from build123d import *

# Parameters (mm, degrees)
F1_DEPTH = 18


with BuildPart() as f1:
    # F0 (on Front) → F1 (new body)
    with BuildSketch(Plane.XZ):
        with BuildLine():
            Line((-494.9431181919, -380.3196549416), (-495.3364644899, -390.3106509103))
            Line((-495.3364644899, -390.3106509103), (-474.3992558025, -390.3106509103))
            Line((-474.3992558025, -390.3106509103), (-442.9078605118, -13.6198989728))
            ThreePointArc((-442.9078605118, -13.6198989728), (-445.4387975319, -5.6995339283), (-438.0486109698, -9.5104350311))
            Line((-438.0486109698, -9.5104350311), (-429.079897486, -10.2602206314))
            ThreePointArc((-429.079897486, -10.2602206314), (-421.1595324415, -7.7292836113), (-424.9704335443, -15.1194701734))
            Line((-424.9704335443, -15.1194701734), (-456.3364644899, -390.3106509103))
            Line((-456.3364644899, -390.3106509103), (-435.3364644899, -390.3106509103))
            Line((-435.3364644899, -390.3106509103), (-349.9298685588, 255.9864675478))
            ThreePointArc((-349.9298685588, 255.9864675478), (-336.6411341811, 280.8261308929), (-310.274619413, 290.7461225986))
            Line((-310.274619413, 290.7461225986), (-55.3364644899, 290.7461225986))
            ThreePointArc((-55.3364644899, 290.7461225986), (-27.0287216569, 302.4853424307), (-15.3365196272, 330.8125378136))
            Line((-15.3365196272, 330.8125378136), (-15.4040666505, 371.4941377938))
            Line((-15.4040666505, 371.4941377938), (-26.1865943467, 371.4941377938))
            Line((-26.1865943467, 371.4941377938), (-26.4555723936, 385.8212303749))
            Line((-26.4555723936, 385.8212303749), (-26.474497292, 389.6893490897))
            Line((-26.474497292, 389.6893490897), (-44.4864644899, 389.6893490897))
            Line((-44.4864644899, 389.6893490897), (-44.4864644899, 371.4941377938))
            Line((-44.4864644899, 371.4941377938), (-55.3364644899, 371.4941377938))
            Line((-55.3364644899, 371.4941377938), (-55.3364644899, 327.1893490897))
            ThreePointArc((-55.3364644899, 327.1893490897), (-57.533163631, 321.8860482309), (-62.8364644899, 319.6893490897))
            ThreePointArc((-62.8364644899, 319.6893490897), (-68.1397653488, 321.8860482309), (-70.3364644899, 327.1893490897))
            Line((-70.3364644899, 327.1893490897), (-70.3364644899, 389.6893490897))
            Line((-70.3364644899, 389.6893490897), (-83.3364644899, 389.6893490897))
            add(Edge.make_bspline(
                [(-83.3364644899, 389.6893490897), (-86.0423866242, 388.9113420461), (-91.2893973468, 387.4027209189), (-94.0159938946, 383.2265543698), (-95.3364644899, 381.2040677155)],
                knots=[0, 0, 0, 0, 0.5157073765, 1, 1, 1, 1], degree=3))
            Line((-95.3364644899, 381.2040677155), (-80.3364644899, 381.2289734555))
            Line((-80.3364644899, 381.2289734555), (-80.3364644899, 327.1893490897))
            ThreePointArc((-80.3364644899, 327.1893490897), (-82.533163631, 321.8860482309), (-87.8364644899, 319.6893490897))
            ThreePointArc((-87.8364644899, 319.6893490897), (-93.1397653488, 321.8860482309), (-95.3364644899, 327.1893490897))
            Line((-95.3364644899, 327.1893490897), (-95.3364644899, 370.6893490897))
            Line((-95.3364644899, 370.6893490897), (-95.3364644899, 371.6893490897))
            Line((-95.3364644899, 371.6893490897), (-435.3364644899, 371.6893490897))
            Line((-435.3364644899, 371.6893490897), (-435.3364644899, 375.1893490897))
            Line((-435.3364644899, 375.1893490897), (-435.3364644899, 376.1893490897))
            Line((-435.3364644899, 376.1893490897), (-435.3364644899, 380.6893490897))
            Line((-435.3364644899, 380.6893490897), (-405.3364644899, 380.6893490897))
            Line((-405.3364644899, 380.6893490897), (-405.3364644899, 389.6893490897))
            Line((-405.3364644899, 389.6893490897), (-445.3364644899, 389.6893490897))
            add(Edge.make_bspline(
                [(-445.3364644899, 389.6893490897), (-450.2049500524, 389.0615823794), (-459.5920285383, 387.2680457186), (-463.5495128465, 378.4364704972), (-465.3198116993, 372.6887939967)],
                knots=[0, 0, 0, 0, 0.4865626406, 1, 1, 1, 1], degree=3))
            Line((-465.3198116993, 372.6887939967), (-465.3905866055, 370.3146473532))
            Line((-465.3905866055, 370.3146473532), (-494.9431181919, -380.3196549416))
        make_face()
    extrude(amount=F1_DEPTH)


solid = f1.part
The listing builds one solid part. Answer for the finished solid, in the listing's coordinates (mm). A direction names the side the tool comes from. Coordinates: 2 decimals unless noted, no trailing zeros. Write each loop counter-clockwise with the first axis right and the second up, starting at its lowest first coordinate (ties: lowest second). Pieces come first, ordered by that corner, then holes. Notation, with made-up numbers: (-32.5, 0) - (-4.5, 0) arc R27 cw to (-4.5, 19) - close; hole circle Ø3 at (-16.5, -21.75). An arc over 180 degrees is marked (long way). Answer as CSV lines item,"result".
1. Determine the mould class of faces 1 (the flat face through (-425, -9, 389.689)), 2 (the flat face through (-393.23, -8.87, -71.69)), 3 (the flat face through (-44.486, -9, 381)) for opening direction X: +X half, -X half, draft (parallel to the pull), parting line (faces both ways), or undercut.
Computed values:
face 1,"draft"
face 2,"+X half"
face 3,"undercut"
2. Given P1, Ø6, axis at y = -4, z = -191.5, coming from the +X side; P2, Ø2.5, axis at y = -9.5, z = 376, coming from the +X side; P3, Ø5.5, axis at x = -20, y = -8.5, coming from the +Z side, each flat-ended and moving along its own axis, determine where each tip first touches the part or whether it passes through.
Computed values:
P1,"stops at x = -408.67"
P2,"stops at x = -26.25"
P3,"stops at z = 371.49"
3. Find section C-C (z = -294.5). Give the vertices of the cut face in (x, y).
Computed values:
outline,"(-491.56, -18) - (-466.39, -18) - (-466.39, 0) - (-491.56, 0) - close; (-448.33, -18) - (-422.68, -18) - (-422.68, 0) - (-448.33, 0) - close"
4. A tool of negligible diameter and unlimited length cuts with its end or side. For faces 4 (the flat face through (-55.336, -9, 350)), 5 (the flat face through (-185, -9, 290.746)), 6 (the flat face through (-80.336, -9, 355)), 7 (the flat face through (-485, -9, -390.311)), from which of +Z, -Z, +X, -X, +Y, -Y can it reach the whole face along a straight path? Write none if from no direction.
Computed values:
face 4,"+Z, +Y, -Y"
face 5,"-Z, +X, +Y, -Y"
face 6,"+Y, -Y"
face 7,"-Z, +X, -X, +Y, -Y"
5. Straight lines are drawn through the part: line 1 (X direction, y = -13, z = -198.5); line 2 (Z direction, x = -179, y = -5.25); line 3 (X direction, y = -7.75, z = -289). For each, find the intervals that lie inside material, in ascending order. Write a range as [from, to].
Computed values:
line 1,"x = [-487.78, -458.36], [-440.3, -409.99]"
line 2,"z = [290.75, 371.69]"
line 3,"x = [-491.35, -465.93], [-447.87, -421.95]"
6. Find section D-D (z = 300). Give the vertices of the cut face in (x, y), plus the area to 3 significant figures.
Computed values:
outline,"(-468.16, -18) - (-29.75, -18) - (-29.75, 0) - (-468.16, 0) - close"
area,"7,890 mm²"
7. Find section A-A (z = -134). Give the vertices of the cut face in (x, y).
Computed values:
outline,"(-485.25, -18) - (-452.97, -18) - (-452.97, 0) - (-485.25, 0) - close; (-434.91, -18) - (-401.47, -18) - (-401.47, 0) - (-434.91, 0) - close"
8. Find section B-B (x = -178.5). Give the vertices of the cut face in (y, z).
Computed values:
outline,"(-18, 290.75) - (0, 290.75) - (0, 371.69) - (-18, 371.69) - close"
